Source: CAD feature listing. Evaluate the final solid. Frame: model axes, mm. Coordinates: 2 decimals unless noted, no trailing zeros. Order: outer loops, then holes, each group sorted by start corner. A loop starts at its lowest first (then second) coordinate and runs counter-clockwise, first axis right, second up. Notation, with made-up numbers: (47, 66.25) -> (72, 66.25) arc R8 ccw to (72, 75.25) -> close; hole circle Ø10 at (67.5, 72). An arc over 180 degrees is marked (long way). Write item = value, one per line. Start each with the question number.
Item 1: Section query D-D (z = -62). Output: boundary loops of the cut face in (x, y), then the cut area to 3 significant figures.
Item 2: Ray query, line 1 along X through (y, z) = (0.5, -34); line 2 along X through (y, z) = (0.45, -12.5); line 3 along X through (y, z) = (1.05, -30.5). Return the intervals inside material, ascending. Write a range as [from, to].
Item 3: Section query B-B (y = 1.3). Output: boundary loops of the cut face in (x, z), then the cut area to 3 significant figures.
Item 4: Section query A-A (x = 9.5). Output: boundary loops of the cut face in (y, z), then the cut area to 3 significant figures.
Item 5: Section query C-C (x = -29.5). Output: boundary loops of the cut face in (y, z).
Item 6: Contact query for a flat-ended pin moving along its axis: pin 1 (3 mm diameter, centred on x = -12, z = -19.5, fed in from +Y). Output: stop coordinate, or through.
```python
from build123d import *

# Parameters (mm, degrees)
BOSS_EXTRUDE1_DEPTH = 1.5875
SKETCH3_W           = 152.4
SKETCH3_H           = 12.7
BOSS_EXTRUDE3_DEPTH = 1.5875
CUT_EXTRUDE1_DEPTH  = 2.5875


with BuildPart() as part:
    # Sketch1 → Boss-Extrude1 (new body)
    with BuildSketch(Plane(origin=(0, 0, 0), x_dir=(1, 0, 0), z_dir=(0, 1, 0))):
        with BuildLine():
            Line((-76.2, 0), (76.2, 0))
            ThreePointArc((76.2, 0), (0, 76.2), (-76.2, 0))
        make_face()
        with BuildLine():
            Line((-12.267257994, 3.287001873), (-36.801773982, 9.861005618))
            ThreePointArc((-36.801773982, 9.861005618), (-29.186293283, 24.490207929), (-16.101755772, 34.530326686))
            Line((-16.101755772, 34.530326686), (-5.367251924, 11.510108895))
            ThreePointArc((-5.367251924, 11.510108895), (-9.728764428, 8.163402643), (-12.267257994, 3.287001873))
        make_face(mode=Mode.SUBTRACT)
        with BuildLine():
            Line((36.801773982, 9.861005619), (12.267257994, 3.287001873))
            ThreePointArc((12.267257994, 3.287001873), (9.728764427, 8.163402643), (5.367251924, 11.510108895))
            Line((5.367251924, 11.510108895), (16.101755772, 34.530326686))
            ThreePointArc((16.101755772, 34.530326686), (29.186293283, 24.490207929), (36.801773982, 9.861005619))
        make_face(mode=Mode.SUBTRACT)
        with BuildLine():
            Line((-13.168222272, 35.752033819), (-5.117344386, 18.486870476))
            ThreePointArc((-5.117344386, 18.486870476), (0, 19.182064372), (5.117344386, 18.486870476))
            Line((5.117344386, 18.486870476), (13.168222272, 35.752033819))
            ThreePointArc((13.168222272, 35.752033819), (0, 38.1), (-13.168222272, 35.752033819))
        make_face(mode=Mode.SUBTRACT)
    extrude(amount=BOSS_EXTRUDE1_DEPTH)

    # Sketch3 → Boss-Extrude3 (add)
    with BuildSketch(Plane(origin=(0, 1.5875, 0), x_dir=(1, 0, 0), z_dir=(0, 1, 0))):
        with Locations((0, -6.35)):
            Rectangle(SKETCH3_W, SKETCH3_H)
    extrude(amount=-BOSS_EXTRUDE3_DEPTH)

    # Sketch4 → Cut-Extrude1 (cut, through all)
    with BuildSketch(Plane(origin=(0, 1.5875, 0), x_dir=(1, 0, 0), z_dir=(0, 1, 0))):
        with BuildLine():
            Line((-1.275735082, 2.15), (-1.275735082, -2.15))
            ThreePointArc((-1.275735082, -2.15), (0, -2.5), (1.275735082, -2.15))
            Line((1.275735082, -2.15), (1.275735082, 2.15))
            ThreePointArc((1.275735082, 2.15), (0, 2.5), (-1.275735082, 2.15))
        make_face()
    extrude(amount=-CUT_EXTRUDE1_DEPTH, mode=Mode.SUBTRACT)


solid = part.part
```
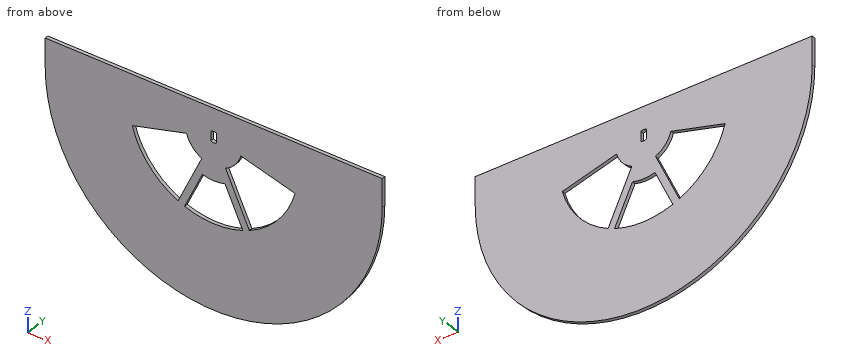
Computed:
q1.outline = (-44.3, 0) -> (44.3, 0) -> (44.3, 1.59) -> (-44.3, 1.59) -> close
q1.area = 141 mm^2
q2.line_1 = [-68.19, -17.19], [-15.85, -12.35], [12.35, 15.85], [17.19, 68.19]
q2.line_2 = [-75.17, -35.99], [-5.83, 5.83], [35.99, 75.17]
q2.line_3 = [-69.83, -22.83], [-14.22, -10.72], [10.72, 14.22], [22.83, 69.83]
q3.outline = (-76.2, 0) arc R76.2 ccw to (76.2, 0) -> (76.2, 12.7) -> (-76.2, 12.7) -> close; hole (-36.8, -9.86) arc R38.1 ccw to (-16.1, -34.53) -> (-5.37, -11.51) arc R12.7 cw to (-12.27, -3.29) -> close; hole (-13.17, -35.75) arc R38.1 ccw to (13.17, -35.75) -> (5.12, -18.49) arc R19.18 cw to (-5.12, -18.49) -> close; hole (-1.28, -2.15) arc R2.5 ccw to (1.28, -2.15) -> (1.28, 2.15) arc R2.5 ccw to (-1.28, 2.15) -> close; hole (5.37, -11.51) -> (16.1, -34.53) arc R38.1 ccw to (36.8, -9.86) -> (12.27, -3.29) arc R12.7 cw to start
q3.area = 9,570 mm^2
q4.outline = (0, -75.61) -> (1.59, -75.61) -> (1.59, -36.9) -> (0, -36.9) -> close; (0, -27.89) -> (1.59, -27.89) -> (1.59, -20.37) -> (0, -20.37) -> close; (0, -8.43) -> (1.59, -8.43) -> (1.59, 12.7) -> (0, 12.7) -> close
q4.area = 107 mm^2
q5.outline = (0, -70.26) -> (1.59, -70.26) -> (1.59, -24.11) -> (0, -24.11) -> close; (0, -7.9) -> (1.59, -7.9) -> (1.59, 12.7) -> (0, 12.7) -> close
q6.pin_1 = through
